Can you work these out from the model? Positions are in its coordinate system, mm. A direction names the side the tool comes from. Coordinates: 2 decimals unless noted, no trailing zeros. Loops run counter-clockwise (first coordinate to the right, second up) from the corner with the lowest first, then second, coordinate; pieces in that order, holes last. Notation, with made-up numbers: M 2.5,-38 L 28.5,-38 A35 ccw 28.5,-3 Z; hole C 9.5,50.25 d11. An arc over 180 degrees is marked long. Answer as a JSON object with one key per item and string values. Group by question number.
Item 1: If I drill on line 1 (Z direction, x = 6.5, y = 2.3); line 2 (X direction, y = 2, z = -5); line 3 (Y direction, x = 5.25, z = -8), over which ranges is the centre line in solid material (lowest first)?
Item 2: Suppose I cut it at B-B (z = -2.25). Write out the boundary of the cut face in (x, y), then the cut area to 3 significant figures.
Item 3: I'm going to push flat-ended pins straight in: pin 1 Ø6 at (y, z) = (47.5, -2.5) entering from +X; pin 2 Ø1.5 at (x, z) = (8, -5) entering from +Y; pin 3 Ø2 at (x, z) = (4.5, -3.5) entering from -Y; pin 4 Ø3.5 at (x, z) = (-2, -6.5) entering from -Y. Where does each tip first touch, or does it pass through?
Item 4: Suppose I cut it at C-C (y = 49.5). Write out the boundary of the cut face in (x, z), then the cut area to 3 significant figures.
Item 5: Which directions (+Z, -Z, +X, -X, +Y, -Y) give clear straight access to the entire face, cutting with the end or side of a thin tool? Please do faces 1 (the flat face through (-1, 62, -5)), 2 (the cylindrical face through (2.86, 3.9, -4.93)).
Item 6: Suppose I cut it at A-A (x = 6.5). Write out the boundary of the cut face in (y, z).
Item 7: We'd pull the mould along X, two halves only. Please class faces 3 (the flat face through (0, 31, -5)), 4 (the cylindrical face through (4.502, 1.542, -5.088)), 5 (the flat face through (9, 3, -5)), 6 (the flat face through (2, 35, -5)): +X half, -X half, draft (parallel to the pull), parting line (faces both ways), or undercut.
Autodesk Inventor part; units mm, degrees
ref_plane "YZ Plane" through (0, 0, 0) normal (1, 0, 0) x (0, 1, 0)
ref_plane "XZ Plane" through (0, 0, 0) normal (0, 1, 0) x (-1, 0, 0)
ref_plane "XY Plane" through (0, 0, 0) normal (0, 0, 1) x (1, 0, 0)
sketch "Sketch1" plane through (0, 0, 0) normal (0, 1, 0) x (-1, 0, 0)
  line L0 (0, 0) -> (-10, 0)
  line L1 (-10, 0) -> (-10, -10)
  line L2 (-10, -10) -> (0, -10)
  line L3 (0, -10) -> (0, 0)
  line L4 (0, 0) -> (-2, 0)
  line L5 (-2, 0) -> (-2, -10)
  dimension "d0" = 10
  dimension "d1" = 10
  dimension "d2" = 2
extrude "Extrusion1" add sketch "Sketch1" along normal blind 3 contours L5 L2 L1 L0
extrude "Extrusion2" add sketch "Sketch1" along normal blind 62 contours L3 L2 L5 L0
sketch "Sketch2" plane through (0, 3, 0) normal (0, 1, 0) x (1, 0, 0)
  line L0 (9.919, 10.0415) -> (10, 5)
  line L1 (10, 0) -> (10, 10)
  line L2 (10, 5) -> (6.5, 5)
  line L3 (2, 0) -> (2, 10)
  circle A0 centre (6.5, 5) radius 2
  point P0 (0, 0)
  dimension "d7" = 3.5
  dimension "d8" = 4
extrude "Extrusion3" cut sketch "Sketch2" against normal blind 62
fillet "Fillet1" radius 3 1 edges at (2, 3, -5)
sketch "Sketch3" plane through (0, 0, -10) normal (-1, 0, 0) x (0, 0, 1)
  line L0 (0, 0) -> (0, 62)
  line L1 (0, 62) -> (0, 66.7685)
  line L2 (0, 66.7685) -> (10, 66.7685)
  line L3 (10, 66.7685) -> (10, 62)
  line L4 (10, 62) -> (0, 62)
  line L5 (10, 62) -> (0, 62)
  point P0 (10, 0)
extrude "Extrusion4" add sketch "Sketch3" along normal blind 3 and the other way blind 2
fillet "Fillet2" radius 2 2 edges at (2, 66.7685, -5) (-3, 66.7685, -5)
properties part number "vacuum_bin_holder" material "Aluminum, Anodized Red"
From the geometry:
{
 "1": {"line 1": "-10 to -7, -3 to 0", "line 2": "0 to 4.5, 8.5 to 10", "line 3": "0 to 3"},
 "2": {"outline": "M -3,62 L 0,62 L 0,0 L 10,0 L 10,3 L 5,3 A3 cw 2,6 L 2,64.77 A2 ccw 0,66.77 L -1,66.77 A2 ccw -3,64.77 Z", "area": "172 mm2"},
 "3": {"pin 1": "x = 2", "pin 2": "y = 3", "pin 3": "y = 0", "pin 4": "y = 62"},
 "4": {"outline": "M 0,-10 L 2,-10 L 2,0 L 0,0 Z", "area": "20.0 mm2"},
 "5": {"face 1": "+Z, -Z, -X, -Y", "face 2": "+Z, -Z, +X, +Y"},
 "6": {"outline": "M 0,-10 L 3,-10 L 3,-7 L 0,-7 Z; M 0,-3 L 3,-3 L 3,0 L 0,0 Z"},
 "7": {"face 3": "-X half", "face 4": "undercut", "face 5": "draft", "face 6": "+X half"}
}
